```python
from build123d import *

# Parameters (mm, degrees)
SKETCH1_W           = 104
SKETCH1_H           = 104
SKETCH1_R           = 21
SKETCH1_R_2         = 4.25
BOSS_EXTRUDE1_DEPTH = 3
SKETCH2_W           = 144
SKETCH2_H           = 144
SKETCH2_W_2         = 104
SKETCH2_H_2         = 104
BOSS_EXTRUDE2_DEPTH = 3


with BuildPart() as part:
    # Sketch1 → Boss-Extrude1 (new body)
    with BuildSketch(Plane.XY):
        Rectangle(SKETCH1_W, SKETCH1_H)
        with Locations((0, 20)):
            Circle(SKETCH1_R, mode=Mode.SUBTRACT)
        with Locations((-42.426406871, 42.426406871)):
            Circle(SKETCH1_R_2, mode=Mode.SUBTRACT)
        with Locations((42.426406871, 42.426406871)):
            Circle(SKETCH1_R_2, mode=Mode.SUBTRACT)
        with Locations((42.426406871, -42.426406871)):
            Circle(SKETCH1_R_2, mode=Mode.SUBTRACT)
        with Locations((-42.426406871, -42.426406871)):
            Circle(SKETCH1_R_2, mode=Mode.SUBTRACT)
    extrude(amount=BOSS_EXTRUDE1_DEPTH)

    # Sketch2 → Boss-Extrude2 (add)
    with BuildSketch(Plane(origin=(0, 0, 0), x_dir=(-1, 0, 0), z_dir=(0, 0, -1))):
        Rectangle(SKETCH2_W, SKETCH2_H)
        Rectangle(SKETCH2_W_2, SKETCH2_H_2, mode=Mode.SUBTRACT)
    extrude(amount=-BOSS_EXTRUDE2_DEPTH)


solid = part.part
```
Part model, mm, in its own coordinate system. Give positions to 0.01 mm unless a question says otherwise; leave off trailing zeros. Write each loop counter-clockwise with the first axis right and the second up, starting at its lowest first coordinate (ties: lowest second). Pieces come first, ordered by that corner, then holes. Notation, with made-up numbers: (87.25, -34.75) -> (119.25, -34.75) arc R23 cw to (119.25, -5.75) -> close; hole circle Ø5 at (51.5, 55.5). An arc over 180 degrees is marked (long way). Put each result on its own line as item: value. Start each with the question number.
Item 1: Cut at A-A (x = 0). List the corners of the cut face in (y, z).
Item 2: Pull direction Y, two halves, no side cores. Call faces 1 (the face through (1, -15, 0)), 2 (the face through (20.03, 26.31, 1.48)): pulls with the +Y half, pulls with the -Y half, needs draft (parallel to the pull), parting line crosses it, or undercut.
Item 3: Cut at B-B (y = 20). List the corners of the cut face in (x, z).
Item 4: Wall check: L1, parallel to Y at x = 43, z = 2.8; L2, parallel to X at y = 41.5, z = 2.45; L3, parallel to Y at x = 0, z = 0.65. Give the ranges that are in metal, low to high. Write a range as [from, to].
Item 5: Cut at C-C (z = 1.65). List the corners of the cut face in (x, y), then the cut area to 3 significant figures.
Answer list:
1. outline: (-72, 0) -> (-1, 0) -> (-1, 3) -> (-72, 3) -> close; (41, 0) -> (72, 0) -> (72, 3) -> (41, 3) -> close
2. face 1: needs draft
2. face 2: undercut
3. outline: (-72, 0) -> (-21, 0) -> (-21, 3) -> (-72, 3) -> close; (21, 0) -> (72, 0) -> (72, 3) -> (21, 3) -> close
4. L1: y = [-72, -46.64], [-38.22, 38.22], [46.64, 72]
4. L2: x = [-72, -46.57], [-38.28, 38.28], [46.57, 72]
4. L3: y = [-72, -1], [41, 72]
5. outline: (-72, -72) -> (72, -72) -> (72, 72) -> (-72, 72) -> close; hole circle Ø8.5 at (-42.43, -42.43); hole circle Ø8.5 at (-42.43, 42.43); hole circle Ø42 at (0, 20); hole circle Ø8.5 at (42.43, -42.43); hole circle Ø8.5 at (42.43, 42.43)
5. area: 19,100 mm2
